Could you check a few things on this model? Use its own coordinates, in mm. A direction names the side the tool comes from. Round coordinates to 2 decimals unless told otherwise and drop trailing zeros. Order: outer loops, then holes, each group sorted by start corner. A loop starts at its lowest first (then second) coordinate and runs counter-clockwise, first axis right, second up. Notation, with made-up numbers: (32, -13.5) -> (79, -13.5) arc R24 ccw to (79, -0.5) -> close; hole circle Ø7 at (31, 9.5). An arc over 180 degrees is marked (long way). Put each result on its own line as item: value. Start each with the question number.
from build123d import *

# Parameters (mm, degrees)
SKETCH1_W           = 75
SKETCH1_H           = 70
BOSS_EXTRUDE1_DEPTH = 4
SKETCH2_W           = 69
SKETCH2_H           = 49
BOSS_EXTRUDE2_DEPTH = 2
SKETCH3_R           = 3
CUT_EXTRUDE1_DEPTH  = 4


with BuildPart() as part:
    # Sketch1 → Boss-Extrude1 (new body)
    with BuildSketch(Plane(origin=(0, 0, 0), x_dir=(1, 0, 0), z_dir=(0, 1, 0))):
        with Locations((12.572182046, -15.652440212)):
            Rectangle(SKETCH1_W, SKETCH1_H)
    extrude(amount=BOSS_EXTRUDE1_DEPTH)

    # Sketch2 → Boss-Extrude2 (add)
    with BuildSketch(Plane(origin=(0, 4, 0), x_dir=(1, 0, 0), z_dir=(0, 1, 0))):
        with Locations((12.572182046, -15.652440212)):
            Rectangle(SKETCH2_W, SKETCH2_H)
    extrude(amount=BOSS_EXTRUDE2_DEPTH)

    # Sketch3 → Cut-Extrude1 (cut)
    with BuildSketch(Plane(origin=(0, 4, 0), x_dir=(1, 0, 0), z_dir=(0, 1, 0))):
        with Locations((12.572182046, 14.347559788)):
            Circle(SKETCH3_R)
        with Locations((12.572182046, -45.652440212)):
            Circle(SKETCH3_R)
    extrude(amount=-CUT_EXTRUDE1_DEPTH, mode=Mode.SUBTRACT)


solid = part.part
1. For pin 1 Ø0.6 at (x, y) = (28.5, 5) entering from +Z; pin 2 Ø1.6 at (y, z) = (5.5, 12.5) entering from -X; pin 3 Ø0.6 at (y, z) = (5, 18) entering from +X, each with a flat end and sliding along its axis, tell me the tip position at first contact or that it passes through.
2. If we section it at D-D, the plane x = 12.5: Please give me the cut outline in (y, z).
3. Which directions (+Z, -Z, +X, -X, +Y, -Y) give clear straight access to the entire face, cutting with the end or side of a thin tool? Please do faces 1 (the face through (47.072, 5, 16)), 2 (the face through (-21.928, 5, 16)), 3 (the face through (12, 5, 40.152)).
4. If we section it at C-C, the plane z = -13.5: Please give me the cut outline in (x, y).
5. If we section it at A-A, the plane z = 27.5: Please give me the cut outline in (x, y).
6. If we section it at B-B, the plane x = -11: Please give me the cut outline in (y, z).
7. Thinking about a two-plate mould opening in Z: for faces 4 (the face through (12, 2, 50.652)), 5 (the face through (15.434, 2.028, 44.751)), 6 (the face through (12, 5, -8.848)), 7 (the face through (15.434, 2.028, -15.249)), which applies, +Z half, -Z half, draft (parallel to the pull), parting line (faces both ways), or undercut?
8. I need wall thicknesses on L1, parallel to Y at x = 36, z = -9; L2, parallel to X at y = 5.65, z = 12; L3, parallel to Z at x = 13, y = 1.55. Which ranges of each line are inside material? Lowest first, please.
Results below:
1. pin 1: z = 40.15
1. pin 2: x = -21.93
1. pin 3: x = 47.07
2. outline: (0, -19.35) -> (4, -19.35) -> (4, -17.35) -> (0, -17.35) -> close; (0, -11.35) -> (4, -11.35) -> (4, -8.85) -> (6, -8.85) -> (6, 40.15) -> (4, 40.15) -> (4, 42.65) -> (0, 42.65) -> close; (0, 48.65) -> (4, 48.65) -> (4, 50.65) -> (0, 50.65) -> close
3. face 1: +Z, -Z, +X, +Y
3. face 2: +Z, -Z, -X, +Y
3. face 3: +Z, +X, -X, +Y
4. outline: (-24.93, 0) -> (9.69, 0) -> (9.69, 4) -> (-24.93, 4) -> close; (15.45, 0) -> (50.07, 0) -> (50.07, 4) -> (15.45, 4) -> close
5. outline: (-24.93, 0) -> (50.07, 0) -> (50.07, 4) -> (47.07, 4) -> (47.07, 6) -> (-21.93, 6) -> (-21.93, 4) -> (-24.93, 4) -> close
6. outline: (0, -19.35) -> (4, -19.35) -> (4, -8.85) -> (6, -8.85) -> (6, 40.15) -> (4, 40.15) -> (4, 50.65) -> (0, 50.65) -> close
7. face 4: +Z half
7. face 5: undercut
7. face 6: -Z half
7. face 7: undercut
8. L1: 0 to 4
8. L2: -21.93 to 47.07
8. L3: -19.35 to -17.32, -11.38 to 42.68, 48.62 to 50.65
